Verification items for the finished model (mm, model axes). Face numbers are marked on the shaded views. A direction names the side the tool comes from. Give positions to 0.01 mm unless a question says otherwise; leave off trailing zeros. Loops run counter-clockwise (first coordinate to the right, second up) from the corner with the lowest first, then second, coordinate; pieces in that order, holes last. Notation, with made-up numbers: (45.5, -16) -> (60.5, -16) arc R30 cw to (60.5, 20) -> close; hole circle Ø7 at (71.25, 5.25). An arc over 180 degrees is marked (long way). Use one line per item in the form item = value. Start each with the question number.
from build123d import *

# Parameters (mm, degrees)
F0_W     = 19.05
F0_H     = 152.4
F1_DEPTH = 31.75
F8_R     = 7.62
F2_DEPTH = 6.35
F3_R     = 4.826
F9_DEPTH = 12.7
F4_R     = 15.87499
F5_DEPTH = 19.05
F8_R_2   = 9.525
F6_DEPTH = 19.05
F7_SIZE  = 0.79375


# Not quite as in the source:
# - a fillet or chamfer is up to 0.001 mm smaller than in the source, because OpenCascade refuses the exact size


with BuildPart() as f1:
    # F0 (on Front) → F1 (new body)
    with BuildSketch(Plane.XZ):
        Rectangle(F0_W, F0_H)
    extrude(amount=F1_DEPTH)

    # F8 (on face) → F2 (cut)
    with BuildSketch(Plane.YZ.offset(9.525)):
        with Locations((-15.875, 60.325)):
            Circle(F8_R)
    extrude(amount=-F2_DEPTH, mode=Mode.SUBTRACT)

    # F3 (on face) → F9 (cut, through all)
    with BuildSketch(Plane.YZ.offset(3.175)):
        with Locations((-15.875, 60.325)):
            Circle(F3_R)
    extrude(amount=-F9_DEPTH, mode=Mode.SUBTRACT)

    # F4 (radius 15.875 in the source; OpenCascade refuses exactly that, so slightly less here)
    f4_edges = [f1.edges().sort_by_distance(p)[0] for p in [
        (0, -31.75, 76.2),
        (0, 0, 76.2),
    ]]
    fillet(f4_edges, radius=F4_R)

    # F8 (on face) → F5 (cut, through all)
    with BuildSketch(Plane.YZ.offset(9.525)):
        Polygon((0, 25.4), (-15.875, 9.525), (0, -6.35), align=None)
    extrude(amount=-F5_DEPTH, mode=Mode.SUBTRACT)

    # F8 (on face) → F6 (cut, through all)
    with BuildSketch(Plane.YZ.offset(9.525)):
        with Locations((-15.875, 34.925)):
            Circle(F8_R_2)
        with Locations((-15.4730585432, -15.8768173255)):
            Circle(F8_R_2)
        with Locations((-15.6740292716, -38.1009086628)):
            Circle(F8_R_2)
        with Locations((-15.875, -60.325)):
            Circle(F8_R_2)
    extrude(amount=-F6_DEPTH, mode=Mode.SUBTRACT)

    # F7
    f7_edges = [f1.edges().sort_by_distance(p)[0] for p in [
        (0, -6.35, 34.925),
        (9.525, -25.4, 34.925),
        (-9.525, -25.4, 34.925),
        (0, -5.948059, -15.876817),
        (9.525, -24.998059, -15.876817),
        (-9.525, -24.998059, -15.876817),
        (0, -6.149029, -38.100909),
        (9.525, -25.199029, -38.100909),
        (-9.525, -25.199029, -38.100909),
        (0, -6.35, -60.325),
        (9.525, -25.4, -60.325),
        (-9.525, -25.4, -60.325),
        (9.525, -23.495, 60.325),
        (-3.175, -11.049, 60.325),
        (3.175, -20.701, 60.325),
        (-9.525, -20.701, 60.325),
    ]]
    chamfer(f7_edges, length=F7_SIZE)


solid = f1.part
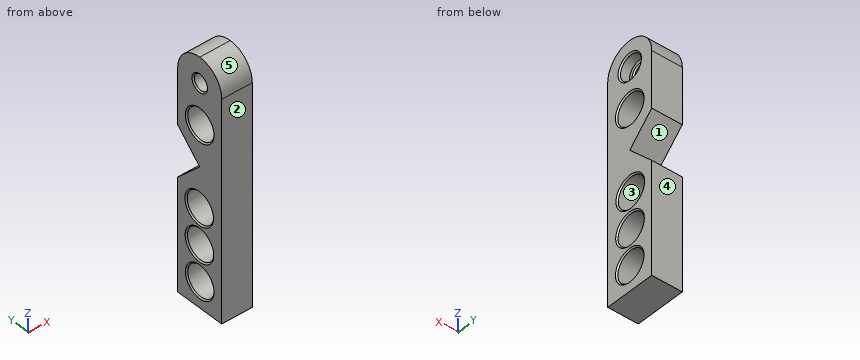
Item 1: Sectioned sample at A-A, the plane x = 5.5. State how many separate pieces and enclosed holes the cut face has, and give its area (3 significant figures).
Item 2: Tool access check on the marked faces 1 and 2. Record the directions out of +Z, -Z, +X, -X, +Y, -Y that give a thin tool (end or side, any length) a straight path to the whole face; none if there is none.
Item 3: Gauge pin test, flat ends, axial feed: pin 1 Ø1.5 at (x, z) = (-5.5, 4) entering from +Y; pin 2 Ø5 at (x, y) = (2, -27.5) entering from +Z. Record the tip position at first contact, or that the pin passes through.
Item 4: Material ranges on line 1 (Y direction, x = 2, z = 35.5); line 2 (Y direction, x = 4.5, z = -68); line 3 (Z direction, x = -5, y = -10.5), recorded low to high.
Item 5: Draft check along Y on the marked faces 3, 4 and 5. Enter one of: +Y half, -Y half, draft (parallel to the pull), parting line (faces both ways), or undercut.
Item 6: Sectioned sample at C-C, the plane z = 19.5. Enter the section's corners in (x, y) (3 decimals).
Outcome:
q1.separate_pieces = 1
q1.enclosed_holes = 5
q1.area = 3,160 mm^2
q2.face_1 = +X, -X, +Y
q2.face_2 = +Z, -Z, +X, -X, -Y
q3.pin_1 = -9.6
q3.pin_2 = 73.32
q4.line_1 = -31.75 to -25.38, -6.37 to 0
q4.line_2 = -31.75 to -21.52, -10.23 to 0
q4.line_3 = -76.2 to -68.19, -52.46 to -46.1, -30.1 to -24, -7.75 to 4.15, 14.9 to 27.06, 42.79 to 75.26
q5.face_3 = undercut
q5.face_4 = +Y half
q5.face_5 = -Y half
q6.outline = (-9.525, -31.75) -> (9.525, -31.75) -> (9.525, -5.9) -> (-9.525, -5.9) -> close
